```python
from build123d import *

# Parameters (mm, degrees)
EXTRUDE_1_DEPTH     = 4
SKETCH_6_R          = 19.5
SKETCH_6_R_2        = 2.6
CUT_EXTRUDE_1_DEPTH = 45.18834688
EXTRUDE_2_DEPTH     = 8
EXTRUDE_3_DEPTH     = 4
EXTRUDE_4_DEPTH     = 4
SKETCH_8_R          = 2.6
CUT_EXTRUDE_2_DEPTH = 137.086222668
SKETCH_12_R         = 5
CUT_EXTRUDE_3_DEPTH = 3
SKETCH_13_R         = 5
CUT_EXTRUDE_4_DEPTH = 0.2
FILLET_1_R          = 2.5
CHAMFER_2_SIZE      = 3


with BuildPart() as part:
    # Эскиз1 → Бобышка-Вытянуть1 (new body)
    with BuildSketch(Plane.XY):
        Polygon((-29, 29), (29, 29), (33.1, 29), (33.1, -29), (29, -29), (-29, -29), align=None)
    extrude(amount=EXTRUDE_1_DEPTH)

    # Эскиз6 → Вырез-Вытянуть1 (cut, through all)
    with BuildSketch(Plane.XY.offset(4)):
        Circle(SKETCH_6_R)
        with Locations((-23.57, 23.57)):
            Circle(SKETCH_6_R_2)
        with Locations((23.57, 23.57)):
            Circle(SKETCH_6_R_2)
        with Locations((-23.57, -23.57)):
            Circle(SKETCH_6_R_2)
        with Locations((23.57, -23.57)):
            Circle(SKETCH_6_R_2)
    extrude(amount=-CUT_EXTRUDE_1_DEPTH, mode=Mode.SUBTRACT)

    # Эскиз3 → Бобышка-Вытянуть2 (add)
    with BuildSketch(Plane(origin=(0, 29, 0), x_dir=(1, 0, 0), z_dir=(0, 1, 0))):
        Polygon((-29, -4), (37.1, -4), (37.1, 108.5), (-2.9, 108.5), (-48.9, 68.5), (-48.9, 28.5), (-29, 28.5), align=None)
    extrude(amount=EXTRUDE_2_DEPTH)

    # Эскиз5 → Бобышка-Вытянуть3 (add)
    with BuildSketch(Plane(origin=(33.1, 0, 0), x_dir=(0, 0, -1), z_dir=(1, 0, 0))):
        Polygon((-4, -29), (-4, 37), (68.5, 37), (68.5, 29), (0, -29), align=None)
    extrude(amount=EXTRUDE_3_DEPTH)

    # Эскиз10 → Бобышка-Вытянуть4 (add)
    with BuildSketch(Plane.ZY.offset(29)):
        Polygon((4, -29), (0, -29), (-68.5, 29), (-68.5, 37), (4, 37), align=None)
    extrude(amount=EXTRUDE_4_DEPTH)

    # Эскиз8 → Вырез-Вытянуть2 (cut, through all)
    with BuildSketch(Plane(origin=(0, 37, 0), x_dir=(1, 0, 0), z_dir=(0, 1, 0))):
        with Locations(Location((27.1, 38.5, 0), (0, 0, 270))):
            Circle(SKETCH_8_R)
        with Locations(Location((7.1, 38.5, 0), (0, 0, 270))):
            Circle(SKETCH_8_R)
        with Locations(Location((7.1, 58.5, 0), (0, 0, 270))):
            Circle(SKETCH_8_R)
        with Locations(Location((7.1, 78.5, 0), (0, 0, 270))):
            Circle(SKETCH_8_R)
        with Locations(Location((7.1, 98.5, 0), (0, 0, 270))):
            Circle(SKETCH_8_R)
        with Locations(Location((27.1, 58.5, 0), (0, 0, 270))):
            Circle(SKETCH_8_R)
        with Locations(Location((27.1, 78.5, 0), (0, 0, 270))):
            Circle(SKETCH_8_R)
        with Locations(Location((27.1, 98.5, 0), (0, 0, 270))):
            Circle(SKETCH_8_R)
        with Locations(Location((-12.9, 58.5, 0), (0, 0, 270))):
            Circle(SKETCH_8_R)
        with Locations(Location((-12.9, 38.5, 0), (0, 0, 270))):
            Circle(SKETCH_8_R)
        with Locations(Location((-38.9, 58.5, 0), (0, 0, 270))):
            Circle(SKETCH_8_R)
        with Locations(Location((-38.9, 38.5, 0), (0, 0, 270))):
            Circle(SKETCH_8_R)
        with Locations(Location((27.1, 18.5, 0), (0, 0, 270))):
            Circle(SKETCH_8_R)
    extrude(amount=-CUT_EXTRUDE_2_DEPTH, mode=Mode.SUBTRACT)

    # Эскиз12 → Вырез-Вытянуть3 (cut)
    with BuildSketch(Plane.XZ.offset(-29)):
        with Locations(Location((27.1, -38.5, 0), (0, 0, 270))):
            Circle(SKETCH_12_R)
        with Locations(Location((7.1, -38.5, 0), (0, 0, 270))):
            Circle(SKETCH_12_R)
        with Locations(Location((-12.9, -38.5, 0), (0, 0, 270))):
            Circle(SKETCH_12_R)
        with Locations(Location((7.1, -58.5, 0), (0, 0, 270))):
            Circle(SKETCH_12_R)
        with Locations(Location((-12.9, -58.5, 0), (0, 0, 270))):
            Circle(SKETCH_12_R)
        with Locations(Location((27.1, -58.5, 0), (0, 0, 270))):
            Circle(SKETCH_12_R)
        with Locations(Location((27.1, -18.5, 0), (0, 0, 270))):
            Circle(SKETCH_12_R)
    extrude(amount=-CUT_EXTRUDE_3_DEPTH, mode=Mode.SUBTRACT)

    # Эскиз13 → Вырез-Вытянуть4 (cut)
    with BuildSketch(Plane.XZ.offset(-29)):
        with Locations(Location((-38.9, -38.5, 0), (0, 0, 270))):
            Circle(SKETCH_13_R)
        with Locations(Location((-38.9, -58.5, 0), (0, 0, 270))):
            Circle(SKETCH_13_R)
        with Locations(Location((27.1, -78.5, 0), (0, 0, 270))):
            Circle(SKETCH_13_R)
        with Locations(Location((7.1, -78.5, 0), (0, 0, 270))):
            Circle(SKETCH_13_R)
        with Locations(Location((7.1, -98.5, 0), (0, 0, 270))):
            Circle(SKETCH_13_R)
        with Locations(Location((27.1, -98.5, 0), (0, 0, 270))):
            Circle(SKETCH_13_R)
    extrude(amount=-CUT_EXTRUDE_4_DEPTH, mode=Mode.SUBTRACT)

    # Скругление1
    fillet_1_edges = [part.edges().sort_by_distance(p)[0] for p in [
        (37.1, 33, -108.5),
        (-2.9, 33, -108.5),
        (-48.9, 33, -68.5),
        (-48.9, 33, -28.5),
        (-33, 33, -28.5),
    ]]
    fillet(fillet_1_edges, radius=FILLET_1_R)

    # Фаска2
    # the kernel refuses this chamfer: 3 mm, written as the material it adds along each edge
    with BuildSketch(Plane(origin=(-29, 29, 0), x_dir=(-0.027495876610586768, -0.9996219169112968, 0), z_dir=(0, 0, -1))) as chamfer_2_piece_1_section:
        Polygon((CHAMFER_2_SIZE * 0.999621916911, -CHAMFER_2_SIZE * 0.0274958766106), (-CHAMFER_2_SIZE * 0.0274958766106, -CHAMFER_2_SIZE * 0.999621916911), (0, 0), align=None)
    chamfer_2_piece_1 = extrude(amount=76.215048964, mode=Mode.PRIVATE)
    chamfer_2_piece_1 = split(chamfer_2_piece_1, bisect_by=Plane(origin=(-27.995614035, 11.406791474, -47.721814069), z_dir=(0, 0.7631749451448332, 0.6461919243562093)), keep=Keep.TOP, mode=Mode.PRIVATE)
    add(chamfer_2_piece_1)
    with BuildSketch(Plane(origin=(33.1, 29, -76.215048964), x_dir=(0.027495876610586768, -0.9996219169112968, 0), z_dir=(0, 0, 1))) as chamfer_2_piece_2_section:
        Polygon((CHAMFER_2_SIZE * 0.999621916911, -CHAMFER_2_SIZE * 0.0274958766106), (-CHAMFER_2_SIZE * 0.0274958766106, -CHAMFER_2_SIZE * 0.999621916911), (0, 0), align=None)
    chamfer_2_piece_2 = extrude(amount=76.215048964, mode=Mode.PRIVATE)
    chamfer_2_piece_2 = chamfer_2_piece_2 - Plane(origin=(27.1, 27.967688512, -58.5), x_dir=(0, 0, -1), z_dir=(0, -1, 0)) * Cylinder(5, 165, mode=Mode.PRIVATE)
    chamfer_2_piece_2 = chamfer_2_piece_2 - Plane(origin=(27.1, 27.967688512, -38.5), x_dir=(0, 0, -1), z_dir=(0, -1, 0)) * Cylinder(5, 165, mode=Mode.PRIVATE)
    chamfer_2_piece_2 = chamfer_2_piece_2 - Plane(origin=(27.1, 27.967688512, -18.5), x_dir=(0, 0, -1), z_dir=(0, -1, 0)) * Cylinder(5, 165, mode=Mode.PRIVATE)
    chamfer_2_piece_2 = split(chamfer_2_piece_2, bisect_by=Plane(origin=(32.179087154, 11.152901074, -47.421960751), z_dir=(0, 0.7631749451448332, 0.6461919243562093)), keep=Keep.TOP, mode=Mode.PRIVATE)
    add(chamfer_2_piece_2)


solid = part.part
```
Read the model definition and answer for the solid it produces. Units are mm, in the model's axes. A direction names the side the tool comes from. Give positions to 0.01 mm unless a question says otherwise; leave off trailing zeros. Order: outer loops, then holes, each group sorted by start corner. A loop starts at its lowest first (then second) coordinate and runs counter-clockwise, first axis right, second up.
(1) For faces 5 (the flat face through (33.1, 11, -18)), 6 (the cylindrical face through (-12.68, 30.479, -53.505)), 7 (the cylindrical face through (-38.8, 33.2, -61.1)), 8 (the cylindrical face through (-2.539, 19.334, 2.028)), 9 (the flat face through (-41, 33, -28.5)), determine the directions among +Z, -Z, +X, -X, +Y, -Y from which every point of the face is accessible in a straight line to the end or side of a thin tool.
(2) Find section B-B (y = 0). Give the vertices of the cut face in (x, z).
(3) Find section C-C (x = -12.9). Give the vertices of the cut face in (y, z), plus the area to 3 significant figures.
(4) Find section A-A (x = 0). Give the vertices of the cut face in (y, z).
(5) Straight lines are drawn through the part: L1, parallel to X at y = 29.1, z = -38.5; L2, parallel to X at y = 35.8, z = -18.5; L3, parallel to X at y = 9.5, z = -17.5. For each, find the intervals that lie inside material, in ascending order.
(6) Find section D-D (y = -23.57). Give the vertices of the cut face in (x, z).
(7) Given pin 1 (6 mm diameter, centred on x = 7.1, z = -78.5, fed in from -Y); pin 2 (4 mm diameter, centred on x = 23.57, y = -23.57, fed in from -Z); pin 3 (11 mm diameter, centred on x = -14.5, z = -58.5, fed in from -Y); pin 4 (1 mm diameter, centred on x = 21.5, y = -12.5, fed in from -Z), each flat-ended and moving along its own axis, determine where each tip first touches the part or whether it passes through.
(8) For a pull along X with two mould halves and no side action, classify faces 1 (the cylindrical face through (-12.68, 30.479, -33.505)), 2 (the flat face through (16, 13, 0)), 3 (the flat face through (3, -29, 2)), 4 (the flat face through (37.1, 19, -27)) as released by +X, released by -X, zero draft, split by the parting line, or undercut.
Result sheet:
1. face 5: -Z, -Y
1. face 6: -Y
1. face 7: +Y, -Y
1. face 8: +Z, -Z
1. face 9: +Z, -X, +Y, -Y
2. outline: (-33, -34.25) - (-29, -34.25) - (-29, 0) - (-19.5, 0) - (-19.5, 4) - (-33, 4) - close; (19.5, 0) - (33.1, 0) - (33.1, -34.25) - (37.1, -34.25) - (37.1, 4) - (19.5, 4) - close
3. outline: (-29, 0) - (-14.62, 0) - (-14.62, 4) - (-29, 4) - close; (14.62, 0) - (29, 0) - (29, -33.5) - (32, -33.5) - (32, -35.9) - (37, -35.9) - (37, 4) - (14.62, 4) - close; (29, -99.8) - (37, -99.8) - (37, -61.1) - (32, -61.1) - (32, -63.5) - (29, -63.5) - close; (29, -53.5) - (32, -53.5) - (32, -55.9) - (37, -55.9) - (37, -41.1) - (32, -41.1) - (32, -43.5) - (29, -43.5) - close
3. area: 833 mm2
4. outline: (-29, 0) - (-19.5, 0) - (-19.5, 4) - (-29, 4) - close; (19.5, 0) - (29, 0) - (29, -108.5) - (37, -108.5) - (37, 4) - (19.5, 4) - close
5. L1: x = -48.9 to -43.9, -33.9 to -17.9, -7.9 to 2.1, 12.1 to 22.1, 32.1 to 37.1
5. L2: x = -33 to 24.5, 29.7 to 37.1
5. L3: x = -33 to -29, 33.1 to 37.1
6. outline: (-33, -6.41) - (-29, -6.41) - (-29, 0) - (-26.17, 0) - (-26.17, 4) - (-33, 4) - close; (-20.97, 0) - (20.97, 0) - (20.97, 4) - (-20.97, 4) - close; (26.17, 0) - (33.1, 0) - (33.1, -6.41) - (37.1, -6.41) - (37.1, 4) - (26.17, 4) - close
7. pin 1: stops at y = 29.2
7. pin 2: passes through
7. pin 3: stops at y = 29
7. pin 4: stops at z = 0
8. face 1: undercut
8. face 2: undercut
8. face 3: zero draft
8. face 4: released by +X
